from build123d import *

# Parameters (mm, degrees)
M4X0_7_TAPPED_HOLE1_D = 3.3


with BuildPart() as part:
    # Sketch2 → Revolve1 (revolve)
    with BuildSketch(Plane(origin=(0, 0, 0), x_dir=(1, 0, 0), z_dir=(0, 1, 0)), mode=Mode.PRIVATE) as revolve1_sk:
        Polygon((7.5, -5), (10, -5), (10, 0), (20, 0), (20, 5), (8.5, 5), (8.5, 2.5), (7.5, 2.5), align=None)
    revolve(revolve1_sk.sketch.rotate(Axis((0, 0, -17.379705215), (0, 0, 1)), 180), axis=Axis((0, 0, -17.379705215), (0, 0, 1)))

    # M4x0.7 Tapped Hole1 (through all)
    with Locations(Plane.XY):
        with Locations((-14.5, 0), (14.5, 0)):
            Hole(M4X0_7_TAPPED_HOLE1_D / 2)


solid = part.part
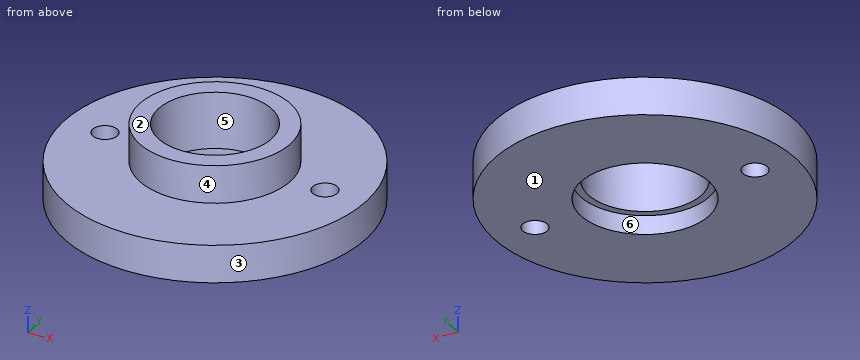
The listing builds one solid part. Answer for the finished solid, in the listing's coordinates (mm). Face numbers are marked on the shaded views. A direction names the side the tool comes from. Give positions to 0.01 mm unless a question says otherwise; leave off trailing zeros. Order: outer loops, then holes, each group sorted by start corner. A loop starts at its lowest first (then second) coordinate and runs counter-clockwise, first axis right, second up. Notation, with made-up numbers: (13, 70.5) - (38, 70.5) arc R25 cw to (38, 87.5) - close; hole circle Ø8 at (60.25, 31.5). An arc over 180 degrees is marked (long way). One line per item, written item: value. Start each with the question number.
1) A cutting plane is placed at D-D on x = 0. Give the vertices of the cut face in (y, z), then the cut area to 3 significant figures.
2) A cutting plane is placed at B-B on x = 14.5. Give the vertices of the cut face in (y, z).
3) The mould has two halves that part along Z. Classify the marked faces 1, 2 and 3: released by +Z, released by -Z, zero draft, split by the parting line, or undercut.
4) A cutting plane is placed at C-C on z = 0.5. Give the vertices of the cut face in (x, y).
5) A tool of negligible diameter and unlimited length cuts with its end or side. For the marked faces 4, 5 and 6, from which of +Z, -Z, +X, -X, +Y, -Y can it reach the whole face along a straight path? Write none if from no direction.
6) Find the intervals of material crossed by L1, parallel to Z at x = 5, y = 16; L2, parallel to Y at x = 0, z = 2.25; L3, parallel to Y at x = -2, z = 2.25, in increasing order.
7) Given pin 1 Ø5 at (x, y) = (11, -9.5) entering from +Z; pin 2 Ø12 at (x, y) = (9, 4.5) entering from +Z; pin 3 Ø2 at (x, y) = (14.5, 0) entering from -Z; pin 4 Ø1.5 at (x, z) = (4.5, 2) entering from -Y, each flat-ended and moving along its own axis, determine where each tip first touches the part or whether it passes through.
8) A cutting plane is placed at A-A on y = 0. Give the vertices of the cut face in (x, z).
Answer sheet:
1. outline: (-20, -5) - (-8.5, -5) - (-8.5, -2.5) - (-7.5, -2.5) - (-7.5, 5) - (-10, 5) - (-10, 0) - (-20, 0) - close; (7.5, -2.5) - (8.5, -2.5) - (8.5, -5) - (20, -5) - (20, 0) - (10, 0) - (10, 5) - (7.5, 5) - close
1. area: 145 mm2
2. outline: (-13.77, -5) - (-1.65, -5) - (-1.65, 0) - (-13.77, 0) - close; (1.65, -5) - (13.77, -5) - (13.77, 0) - (1.65, 0) - close
3. face 1: released by -Z
3. face 2: released by +Z
3. face 3: zero draft
4. outline: circle Ø20 at (0, 0); hole circle Ø15 at (0, 0)
5. face 4: +Z
5. face 5: +Z, -Z
5. face 6: -Z
6. L1: z = -5 to 0
6. L2: y = -10 to -7.5, 7.5 to 10
6. L3: y = -9.8 to -7.23, 7.23 to 9.8
7. pin 1: stops at z = 0
7. pin 2: stops at z = 5
7. pin 3: passes through
7. pin 4: stops at y = -9.27
8. outline: (-20, -5) - (-16.15, -5) - (-16.15, 0) - (-20, 0) - close; (-12.85, -5) - (-8.5, -5) - (-8.5, -2.5) - (-7.5, -2.5) - (-7.5, 5) - (-10, 5) - (-10, 0) - (-12.85, 0) - close; (7.5, -2.5) - (8.5, -2.5) - (8.5, -5) - (12.85, -5) - (12.85, 0) - (10, 0) - (10, 5) - (7.5, 5) - close; (16.15, -5) - (20, -5) - (20, 0) - (16.15, 0) - close
